from build123d import *

# Parameters (mm, degrees)
SKETCH1_W                       = 64
SKETCH1_H                       = 40
BOSS_EXTRUDE1_DEPTH             = 2
SKETCH2_W                       = 2
SKETCH2_H                       = 40
BOSS_EXTRUDE2_DEPTH             = 16
SKETCH3_R                       = 2
CUT_EXTRUDE1_DEPTH              = 78.149206088
LPATTERN1_COUNT                 = 7
LPATTERN1_PITCH                 = 8
MIRROR1_COPY_1_SKETCH_R         = 2
MIRROR1_COPY_1_DEPTH            = 78.149206088
MIRROR1_COPY_2_SKETCH_R         = 2
MIRROR1_COPY_2_DEPTH            = 78.149206088
MIRROR1_COPY_3_SKETCH_R         = 2
MIRROR1_COPY_3_DEPTH            = 78.149206088
MIRROR1_COPY_4_SKETCH_R         = 2
MIRROR1_COPY_4_DEPTH            = 78.149206088
MIRROR1_COPY_5_SKETCH_R         = 2
MIRROR1_COPY_5_DEPTH            = 78.149206088
MIRROR1_COPY_6_SKETCH_R         = 2
MIRROR1_COPY_6_DEPTH            = 78.149206088
CUT_EXTRUDE2_DEPTH              = 78.149206088
TAP_DRILL_FOR_M4X0_7_TAP1_D     = 3.3
TAP_DRILL_FOR_M4X0_7_TAP1_DEPTH = 10.76
SKETCH7_R                       = 2.05
CUT_EXTRUDE3_DEPTH              = 76.947350184
LPATTERN2_COUNT                 = 5
LPATTERN2_PITCH                 = 8
LPATTERN2_COUNT_DIR2            = 2
LPATTERN2_PITCH_DIR2            = 8
FILLET1_R                       = 2


with BuildPart() as part:
    # Sketch1 → Boss-Extrude1 (new body)
    with BuildSketch(Plane(origin=(0, 0, 0), x_dir=(1, 0, 0), z_dir=(0, 1, 0))):
        with Locations((32, 20)):
            Rectangle(SKETCH1_W, SKETCH1_H)
    extrude(amount=BOSS_EXTRUDE1_DEPTH)

    # Sketch2 → Boss-Extrude2 (add)
    with BuildSketch(Plane(origin=(0, 2, 0), x_dir=(1, 0, 0), z_dir=(0, 1, 0))):
        with Locations((1, 20)):
            Rectangle(SKETCH2_W, SKETCH2_H)
    extrude(amount=BOSS_EXTRUDE2_DEPTH)

    # Sketch3 → Cut-Extrude1 (cut, through all)
    with BuildSketch(Plane(origin=(0, 2, 0), x_dir=(1, 0, 0), z_dir=(0, 1, 0))):
        with Locations(Location((8, 36, 0), (0, 0, 270))):
            Circle(SKETCH3_R)
    cut_extrude1 = extrude(amount=-CUT_EXTRUDE1_DEPTH, mode=Mode.SUBTRACT)

    # LPattern1: Cut-Extrude1 ×7
    with Locations(*[(i * LPATTERN1_PITCH, 0, 0) for i in range(1, LPATTERN1_COUNT)]):
        add(cut_extrude1, mode=Mode.SUBTRACT)

    # Mirror1: Cut-Extrude1 across plane
    add(cut_extrude1.mirror(Plane(origin=(0, 0, -20), x_dir=(1, 0, 0), z_dir=(0, 0, -1))), mode=Mode.SUBTRACT)

    # Mirror1 copy 1 sketch → Mirror1 copy 1 (cut, through all)
    with BuildSketch(Plane(origin=(8, 2, -40), x_dir=(1, 0, 0), z_dir=(0, 1, 0))):
        with Locations((8, -36)):
            Circle(MIRROR1_COPY_1_SKETCH_R)
    extrude(amount=-MIRROR1_COPY_1_DEPTH, mode=Mode.SUBTRACT)

    # Mirror1 copy 2 sketch → Mirror1 copy 2 (cut, through all)
    with BuildSketch(Plane(origin=(16, 2, -40), x_dir=(1, 0, 0), z_dir=(0, 1, 0))):
        with Locations((8, -36)):
            Circle(MIRROR1_COPY_2_SKETCH_R)
    extrude(amount=-MIRROR1_COPY_2_DEPTH, mode=Mode.SUBTRACT)

    # Mirror1 copy 3 sketch → Mirror1 copy 3 (cut, through all)
    with BuildSketch(Plane(origin=(24, 2, -40), x_dir=(1, 0, 0), z_dir=(0, 1, 0))):
        with Locations((8, -36)):
            Circle(MIRROR1_COPY_3_SKETCH_R)
    extrude(amount=-MIRROR1_COPY_3_DEPTH, mode=Mode.SUBTRACT)

    # Mirror1 copy 4 sketch → Mirror1 copy 4 (cut, through all)
    with BuildSketch(Plane(origin=(32, 2, -40), x_dir=(1, 0, 0), z_dir=(0, 1, 0))):
        with Locations((8, -36)):
            Circle(MIRROR1_COPY_4_SKETCH_R)
    extrude(amount=-MIRROR1_COPY_4_DEPTH, mode=Mode.SUBTRACT)

    # Mirror1 copy 5 sketch → Mirror1 copy 5 (cut, through all)
    with BuildSketch(Plane(origin=(40, 2, -40), x_dir=(1, 0, 0), z_dir=(0, 1, 0))):
        with Locations((8, -36)):
            Circle(MIRROR1_COPY_5_SKETCH_R)
    extrude(amount=-MIRROR1_COPY_5_DEPTH, mode=Mode.SUBTRACT)

    # Mirror1 copy 6 sketch → Mirror1 copy 6 (cut, through all)
    with BuildSketch(Plane(origin=(48, 2, -40), x_dir=(1, 0, 0), z_dir=(0, 1, 0))):
        with Locations((8, -36)):
            Circle(MIRROR1_COPY_6_SKETCH_R)
    extrude(amount=-MIRROR1_COPY_6_DEPTH, mode=Mode.SUBTRACT)

    # Sketch4 → Cut-Extrude2 (cut, through all)
    with BuildSketch(Plane(origin=(0, 2, 0), x_dir=(1, 0, 0), z_dir=(0, 1, 0))):
        with BuildLine():
            Line((13.2, 30.4), (54.8, 30.4))
            Line((54.8, 30.4), (54.8, 26.2))
            ThreePointArc((54.8, 26.2), (56.030151519, 23.230151519), (59, 22))
            ThreePointArc((59, 22), (61, 20), (59, 18))
            ThreePointArc((59, 18), (56.030151519, 16.769848481), (54.8, 13.8))
            Line((54.8, 13.8), (54.8, 9.6))
            Line((54.8, 9.6), (13.2, 9.6))
            Line((13.2, 9.6), (13.2, 13.8))
            ThreePointArc((13.2, 13.8), (11.969848481, 16.769848481), (9, 18))
            ThreePointArc((9, 18), (7, 20), (9, 22))
            ThreePointArc((9, 22), (11.969848481, 23.230151519), (13.2, 26.2))
            Line((13.2, 26.2), (13.2, 30.4))
        make_face()
    extrude(amount=-CUT_EXTRUDE2_DEPTH, mode=Mode.SUBTRACT)

    # Tap Drill for M4x0.7 Tap1
    with Locations(Plane(origin=(0, 2, 0), x_dir=(1, 0, 0), z_dir=(0, 1, 0))):
        with Locations((9, 25), (9, 15), (59, 15), (59, 25)):
            Hole(TAP_DRILL_FOR_M4X0_7_TAP1_D / 2, depth=TAP_DRILL_FOR_M4X0_7_TAP1_DEPTH)

    # Sketch7 → Cut-Extrude3 (cut, through all)
    with BuildSketch(Plane(origin=(2, 0, 0), x_dir=(0, 0, -1), z_dir=(1, 0, 0))):
        with Locations((4, 14)):
            Circle(SKETCH7_R)
    cut_extrude3 = extrude(amount=-CUT_EXTRUDE3_DEPTH, mode=Mode.SUBTRACT)

    # LPattern2: Cut-Extrude3 5 × 2
    with Locations(*[(0, -j * LPATTERN2_PITCH_DIR2, -i * LPATTERN2_PITCH) for i in range(LPATTERN2_COUNT) for j in range(LPATTERN2_COUNT_DIR2) if (i, j) != (0, 0)]):
        add(cut_extrude3, mode=Mode.SUBTRACT)

    # Fillet1
    fillet1_edges = [part.edges().sort_by_distance(p)[0] for p in [
        (1, 18, 0),
        (1, 18, -40),
        (0, 0, -20),
        (64, 1, -40),
        (64, 1, 0),
    ]]
    fillet(fillet1_edges, radius=FILLET1_R)


solid = part.part
Could you check a few things on this model? Use its own coordinates, in mm. A direction names the side the tool comes from. Round coordinates to 2 decimals unless told otherwise and drop trailing zeros. Loops run counter-clockwise (first coordinate to the right, second up) from the corner with the lowest first, then second, coordinate; pieces in that order, holes last. Notation, with made-up numbers: (51.5, 64) -> (67.5, 64) arc R35 ccw to (67.5, 101) -> close; hole circle Ø11 at (-33, -17.75). An arc over 180 degrees is marked (long way). Use CSV: the item, a comma, the result in double quotes.
(1) Suppose I cut it at B-B on z = -20. Write out the boundary of the cut face in (x, y), plus the area to 3 significant figures.
Return value:
outline,"(0, 2) arc R2 ccw to (2, 0) -> (7, 0) -> (7, 2) -> (2, 2) -> (2, 3.95) -> (0, 3.95) -> close; (0, 8.05) -> (2, 8.05) -> (2, 11.95) -> (0, 11.95) -> close; (0, 16.05) -> (2, 16.05) -> (2, 18) -> (0, 18) -> close; (61, 0) -> (64, 0) -> (64, 2) -> (61, 2) -> close"
area,"34.7 mm²"
(2) For faces 1 (the cylindrical face through (1.014, 12.753, -10.373)), 2 (the flat face through (13.2, 1, -28)), which set-ups out of +Z, -Z, +X, -X, +Y, -Y let a thin tool reach every point of the face, with its end or its side?
Return value:
face 1,"+X, -X"
face 2,"+Y, -Y"
(3) If we mould it in two halves opening along Z, with no side actions, what happens to faces 3 (the cylindrical face through (1.01, 17.43, -39.4)), 4 (the flat face through (26, 2, -34)), 5 (the flat face through (34, 1, -9.6))? For each: +Z half, -Z half, draft (parallel to the pull), parting line (faces both ways), or undercut.
Return value:
face 3,"-Z half"
face 4,"draft"
face 5,"undercut"
(4) Suppose I cut it at C-C on z = -33. Write out the boundary of the cut face in (x, y).
Return value:
outline,"(0, 2) arc R2 ccw to (2, 0) -> (64, 0) -> (64, 2) -> (2, 2) -> (2, 18) -> (0, 18) -> close"
(5) Suppose I cut it at A-A on x = 44. Write out the boundary of the cut face in (y, z).
Return value:
outline,"(0, -40) -> (2, -40) -> (2, -30.4) -> (0, -30.4) -> close; (0, -9.6) -> (2, -9.6) -> (2, 0) -> (0, 0) -> close"
(6) Will these pins go through, and if not, where does the flat tip stop? pin 1 Ø4.5 at (y, z) = (14, -12) entering from +X; pin 2 Ø5.5 at (x, z) = (9, -15) entering from +Y.
Return value:
pin 1,"stops at x = 2"
pin 2,"stops at y = 2"
(7) Suppose I cut it at D-D on z = -25. Write out the boundary of the cut face in (x, y).
Return value:
outline,"(0, 2) arc R2 ccw to (2, 0) -> (7.35, 0) -> (7.35, 2) -> (2, 2) -> (2, 18) -> (0, 18) -> close; (10.65, 0) -> (13.02, 0) -> (13.02, 2) -> (10.65, 2) -> close; (54.98, 0) -> (57.35, 0) -> (57.35, 2) -> (54.98, 2) -> close; (60.65, 0) -> (64, 0) -> (64, 2) -> (60.65, 2) -> close"
(8) If I drill on probe 1 along Y at (x, z) = (0.75, -28); probe 2 along Y at (x, z) = (56.5, -15); probe 3 along Z at (x, y) = (31, 1), over which ranges is the centre line in solid material (lowest first)? Write a range as [from, to].
Return value:
probe 1,"y = [0.44, 3.95], [8.05, 11.95], [16.05, 18]"
probe 2,"y = [0, 2]"
probe 3,"z = [-40, -37.73], [-34.27, -30.4], [-9.6, -5.73], [-2.27, 0]"
